Drawing for the job (mm, zero at the part's lowest x, y, z). A direction names the side the tool comes from. Give positions to 0.01 mm unless a question says otherwise; leave off trailing zeros. Loops run counter-clockwise (first coordinate to the right, second up) from the corner with the lowest first, then second, coordinate; pieces in that order, holes last. Notation, with made-up numbers: (-10.75, 24) - (18.25, 24) arc R8 cw to (18.25, 37) - close; hole circle Ø3 at (57, 70). An arc over 180 degrees is marked (long way). Return JSON: item names as keys, results as strings. Group by question number.
1) Mould opens along Z. For the marked faces 1, 2 and 3 say: released by +Z, released by -Z, zero draft, split by the parting line, or undercut.
2) Drop flat-ended pins along their axis: pin 1 (12 mm diameter, centred on x = 404.5, y = 461.5, fed in from +Z); pin 2 (1 mm diameter, centred on x = 224, y = 285.5, fed in from +Z); pin 3 (3 mm diameter, centred on x = 324.5, y = 717.5, fed in from +Z). Give the stop position or say it passes through.
3) Slice it at C-C (x = 148). List the corners of the cut face in (y, z).
4) 3-axis set-ups, long thin cutter, end or side, ignore diameter. For the marked faces 4 and 5: which of +Z, -Z, +X, -X, +Y, -Y reach the whole face in a straight line?
5) Slice it at B-B (z = 307.5). List the corners of the cut face in (x, y), and give its area (3 significant figures).
6) Drill centre lines: probe 1 along X at (y, z) = (619, 109); probe 2 along Z at (x, y) = (234, 642); probe 3 along Z at (x, y) = (494, 338). Where is each one in solid material? Low to high. Write a range as from..to.
7) Slice it at A-A (y = 719). List the corners of the cut face in (x, z) (1 decimal), and give its area (3 significant figures).
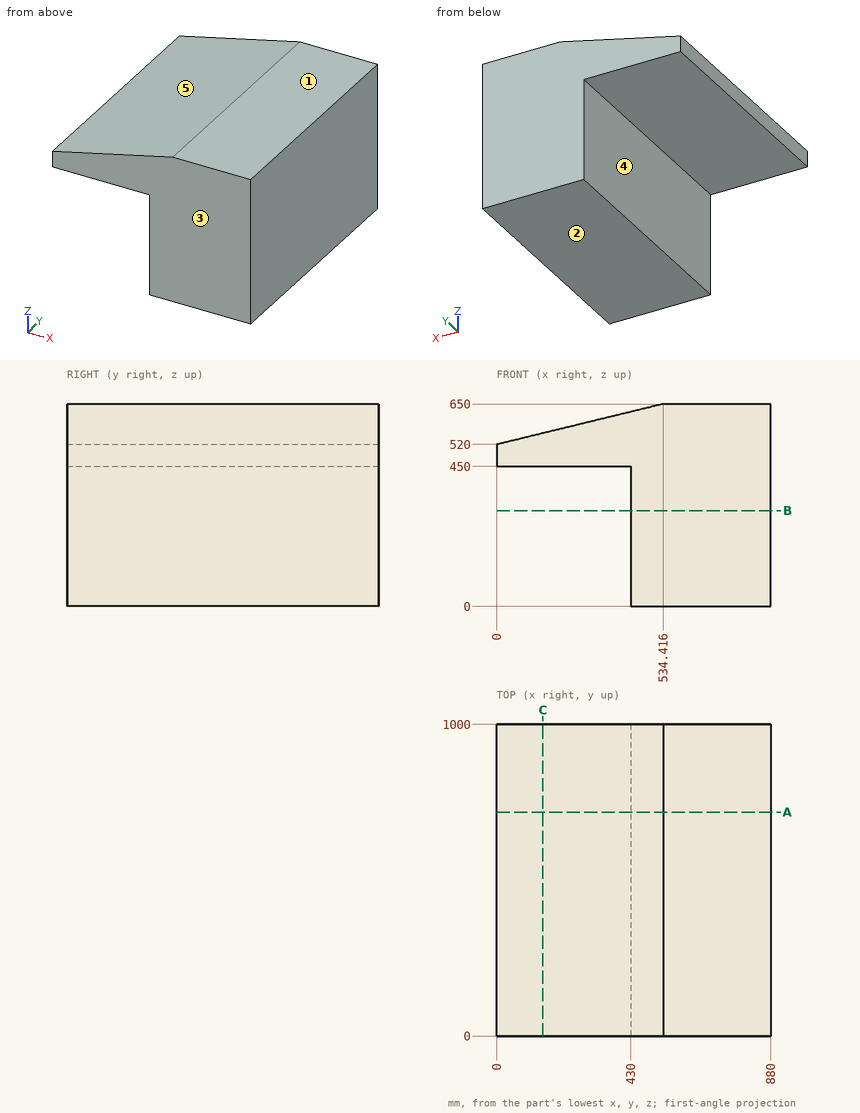
Results:
{
 "1": {"face 1": "released by +Z", "face 2": "released by -Z", "face 3": "zero draft"},
 "2": {"pin 1": "z = 619.86", "pin 2": "z = 574.61", "pin 3": "z = 599.3"},
 "3": {"outline": "(0, 450) - (1000, 450) - (1000, 556) - (0, 556) - close"},
 "4": {"face 4": "-Z, -X, +Y, -Y", "face 5": "+Z, -X, +Y, -Y"},
 "5": {"outline": "(430, 0) - (880, 0) - (880, 1000) - (430, 1000) - close", "area": "450,000 mm2"},
 "6": {"probe 1": "430..880", "probe 2": "450..576.92", "probe 3": "0..640.17"},
 "7": {"outline": "(0, 450) - (430, 450) - (430, 0) - (880, 0) - (880, 650) - (534.4, 650) - (0, 520) - close", "area": "344,000 mm2"}
}
